from build123d import *

# Parameters (mm, degrees)
BOSS_EXTRU_1_DEPTH      = 8.5
CONG_2_R                = 2
ESQUISSE2_R             = 3
ENL_V_MAT_EXTRU_1_DEPTH = 65.453547263
COQUE3_START            = 1.5
COQUE3_DEPTH            = 7


# Read off the part's stored shape, not the designer's step: Coque3
with BuildPart() as part:
    # Esquisse1 → Boss.-Extru.1 (new body)
    with BuildSketch(Plane(origin=(0, 0, 0), x_dir=(1, 0, 0), z_dir=(0, 1, 0))):
        with BuildLine():
            Line((-12.25, 0), (0, -72.75))
            Line((0, -72.75), (12.25, 0))
            ThreePointArc((12.25, 0), (0, 12.25), (-12.25, 0))
        make_face()
    extrude(amount=BOSS_EXTRU_1_DEPTH)

    # Congé2
    cong_2_edges = [part.edges().sort_by_distance(p)[0] for p in [
        (0, 4.25, 72.75),
    ]]
    fillet(cong_2_edges, radius=CONG_2_R)

    # Esquisse2 → Enlèv. mat.-Extru.1 (cut, through all)
    with BuildSketch(Plane(origin=(0, 8.5, 0), x_dir=(1, 0, 0), z_dir=(0, 1, 0))):
        with Locations(Location((-6.25, 0, 0), (0, 0, 270))):
            Circle(ESQUISSE2_R)
        with Locations(Location((4.25, 0, 0), (0, 0, 270))):
            Circle(ESQUISSE2_R)
    extrude(amount=-ENL_V_MAT_EXTRU_1_DEPTH, mode=Mode.SUBTRACT)

    # Coque3 outline → Coque3 (cut)
    with BuildSketch(Plane(origin=(0, 0, 0), x_dir=(1, 0, 0), z_dir=(0, 1, 0)).offset(COQUE3_START)):
        with BuildLine():
            ThreePointArc((7.955882353, 4.718732455), (0.74891051, 9.219633021), (-7.09, 5.940909021))
            ThreePointArc((-7.09, 5.940909021), (-3.572947636, 5.369673234), (-1, 2.90473751))
            ThreePointArc((-1, 2.90473751), (3.058899986, 5.880585069), (7.955882353, 4.718732455))
        make_face()
        with BuildLine():
            ThreePointArc((8.493518341, -4.241762852), (3.413244048, -5.941366802), (-1, -2.90473751))
            ThreePointArc((-1, -2.90473751), (-4.123405548, -5.610489821), (-8.255570494, -5.654881696))
            Line((-8.255570494, -5.654881696), (0, -54.68286157))
            Line((0, -54.68286157), (8.493518341, -4.241762852))
        make_face()
    extrude(amount=COQUE3_DEPTH, mode=Mode.SUBTRACT)

    # Symétrie3: part across plane


with BuildPart() as part_1:
    add(part.part)
    add(part.part.mirror(Plane(origin=(0, 0, 0), x_dir=(0, 0, 1), z_dir=(0, -1, 0))))


solid = part_1.part
CAD build for the part. Positions are in the model's coordinates, mm. A direction names the side the tool comes from. Coordinates: 2 decimals unless noted, no trailing zeros. Order: outer loops, then holes, each group sorted by start corner. A loop starts at its lowest first (then second) coordinate and runs counter-clockwise, first axis right, second up.
Item 1: Pin check, flat tips, straight feed: pin 1 Ø4 at (y, z) = (-5, 44) entering from +X; pin 2 Ø1 at (x, y) = (-5.5, 0.5) entering from -Z; pin 3 Ø3 at (x, z) = (0, -7.5) entering from +Y. Stop position of each tip, or through.
Check sheet entries:
pin 1: stops at x = 5.18
pin 2: stops at z = -11.18
pin 3: stops at y = 1.5
Item 2: Drill centre lines: L1, parallel to X at y = 3, z = 0; L2, parallel to X at y = -7, z = 17.5; L3, parallel to X at y = -5, z = 39. Where is each one in solid material? Low to high.
Check sheet entries:
L1: x = -12.25 to -9.25, -3.25 to 1.25, 7.25 to 12.25
L2: x = -9.3 to -6.26, 6.26 to 9.3
L3: x = -5.68 to -2.64, 2.64 to 5.68
Item 3: Band-saw the part on D-D on y = -5.5. List the corners of the cut face in (x, z), plus the area to 3 significant figures.
Check sheet entries:
outline: (-12.25, 0) arc R12.25 ccw to (12.25, 0) - (1.97, 61.04) arc R2 ccw to (-1.97, 61.04) - close; hole circle Ø6 at (-6.25, 0); hole (-8.26, 5.65) arc R6 cw to (-1, 2.9) arc R6 cw to (8.49, 4.24) - (0, 54.68) - close; hole (-7.09, -5.94) arc R9.25 ccw to (7.96, -4.72) arc R6 cw to (-1, -2.9) arc R6 cw to start; hole circle Ø6 at (4.25, 0)
area: 599 mm2
Item 4: Two-plate mould, pull along Z, no slides. Class faces 1 (the face through (7.04, 0.12, 30.95)), 2 (the face through (2.988, -4.951, -5.866)), 3 (the face through (-6, -8.5, 20)): +Z half, -Z half, draft (parallel to the pull), parting line (faces both ways), or undercut.
Check sheet entries:
face 1: +Z half
face 2: undercut
face 3: draft
Item 5: Band-saw the part on C-C on z = 53. List the corners of the cut face in (x, y).
Check sheet entries:
outline: (-3.33, -8.5) - (-0.28, -8.5) - (-0.28, -1.5) - (0.28, -1.5) - (0.28, -8.5) - (3.33, -8.5) - (3.33, 8.5) - (0.28, 8.5) - (0.28, 1.5) - (-0.28, 1.5) - (-0.28, 8.5) - (-3.33, 8.5) - close
Item 6: Band-saw the part on A-A on z = -1. List the corners of the cut face in (x, y).
Check sheet entries:
outline: (-12.21, -8.5) - (-9.08, -8.5) - (-9.08, 8.5) - (-12.21, 8.5) - close; (-3.42, -8.5) - (1.42, -8.5) - (1.42, 8.5) - (-3.42, 8.5) - close; (7.08, -8.5) - (12.21, -8.5) - (12.21, 8.5) - (7.08, 8.5) - close
Item 7: 3-axis set-ups, long thin cutter, end or side, ignore diameter. For faces 4 (the face through (-6, 8.5, 20)), 5 (the face through (4.187, -4.951, 29.815)), 6 (the face through (-4.186, 4.951, 29.826)): which of +Z, -Z, +X, -X, +Y, -Y reach the whole face in a straight line?
Check sheet entries:
face 4: +Z, -Z, +X, -X, +Y
face 5: -Y
face 6: +Y
Item 8: Band-saw the part on B-B on x = -6.25. List the corners of the cut face in (y, z).
Check sheet entries:
outline: (-8.5, -10.54) - (8.5, -10.54) - (8.5, -6.82) - (1.5, -6.82) - (1.5, -6) - (8.5, -6) - (8.5, -3) - (-8.5, -3) - (-8.5, -6) - (-1.5, -6) - (-1.5, -6.82) - (-8.5, -6.82) - close; (-8.5, 3) - (8.5, 3) - (8.5, 6) - (1.5, 6) - (1.5, 17.57) - (8.5, 17.57) - (8.5, 35.63) - (-8.5, 35.63) - (-8.5, 17.57) - (-1.5, 17.57) - (-1.5, 6) - (-8.5, 6) - close
